The model under review builds one solid part; all positions refer to its coordinate system, in mm. Face numbers are marked on the shaded views. A direction names the side the tool comes from. Coordinates: 2 decimals unless noted, no trailing zeros. Order: outer loops, then holes, each group sorted by start corner. A loop starts at its lowest first (then second) coordinate and runs counter-clockwise, first axis right, second up. Notation, with made-up numbers: (-10.5, 3.5) -> (43.5, 3.5) arc R9 ccw to (43.5, 16.5) -> close; hole circle Ø4 at (6, -8.5). An arc over 180 degrees is marked (long way). Answer as CSV lines item,"result". Start each with the question number.
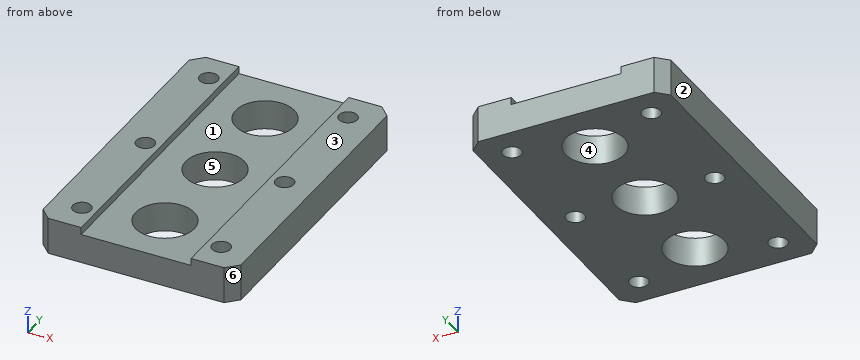
from build123d import *

# Parameters (mm, degrees)
F0_W     = 54
F0_H     = 82
F0_R     = 2.5
F0_R_2   = 8
F1_DEPTH = 10
F2_SIZE  = 3
F3_W     = 30
F3_H     = 82
F4_DEPTH = 2
F5_R     = 8
F6_DEPTH = 25


with BuildPart() as f1:
    # F0 (on Top) → F1 (new body)
    with BuildSketch(Plane.XY):
        Rectangle(F0_W, F0_H)
        with Locations((-19, -33)):
            Circle(F0_R, mode=Mode.SUBTRACT)
        with Locations((0, -26)):
            Circle(F0_R_2, mode=Mode.SUBTRACT)
        with Locations((19, -33)):
            Circle(F0_R, mode=Mode.SUBTRACT)
        with Locations((-19, 0)):
            Circle(F0_R, mode=Mode.SUBTRACT)
        with Locations((-19, 33)):
            Circle(F0_R, mode=Mode.SUBTRACT)
        with Locations((19, 0)):
            Circle(F0_R, mode=Mode.SUBTRACT)
        with Locations((0, 26)):
            Circle(F0_R_2, mode=Mode.SUBTRACT)
        with Locations((19, 33)):
            Circle(F0_R, mode=Mode.SUBTRACT)
    extrude(amount=F1_DEPTH)

    # F2
    f2_edges = [f1.edges().sort_by_distance(p)[0] for p in [
        (27, -41, 5),
        (-27, -41, 5),
        (27, 41, 5),
        (-27, 41, 5),
    ]]
    chamfer(f2_edges, length=F2_SIZE)

    # F3 (on face) → F4 (cut)
    with BuildSketch(Plane.XY.offset(10)):
        Rectangle(F3_W, F3_H)
    extrude(amount=-F4_DEPTH, mode=Mode.SUBTRACT)

    # F5 (on face) → F6 (cut)
    with BuildSketch(Plane.XY.offset(8)):
        Circle(F5_R)
    extrude(amount=-F6_DEPTH, mode=Mode.SUBTRACT)


solid = f1.part
1) Insertion check: pin 1 Ø9.5 at (x, y) = (0, 0) entering from -Z; pin 2 Ø1 at (x, y) = (10.5, 28) entering from +Z. Each pin has a flat end and moves straight along its axis. Give the tip position at first contact, or say it passes through.
2) Consider section B-B (x = -19). Give the boundary of the cut face in (y, z), plus the area to 3 significant figures.
3) Tool access review of the marked faces 1 and 2: name each direction out of +Z, -Z, +X, -X, +Y, -Y from which nothing blocks a thin tool from reaching the whole face with its end or side.
4) Consider section D-D (z = 1). Count the separate pieces of the cut face and the enclosed holes in it, plus the area to 3 significant figures.
5) Consider section C-C (y = -26). Give the boundary of the cut face in (x, z).
6) Mouldability with a two-part tool opening along Y and no side actions: class the marked faces 3, 4, 5 and 6 as released by +Y, released by -Y, zero draft, split by the parting line, or undercut.
7) Consider section A-A (z = 9). Give the boundary of the cut face in (x, y).
8) Wall thickness on L1, parallel to Y at x = -19, z = 2.5; L2, parallel to Y at x = 0, z = 6; L3, parallel to X at y = 26, z = 3.75: over which ranges is each line inside the solid? List them lowest first. Write a range as [from, to].
Result:
1,pin 1,"through"
1,pin 2,"z = 8"
2,outline,"(-41, 0) -> (-35.5, 0) -> (-35.5, 10) -> (-41, 10) -> close; (-30.5, 0) -> (-2.5, 0) -> (-2.5, 10) -> (-30.5, 10) -> close; (2.5, 0) -> (30.5, 0) -> (30.5, 10) -> (2.5, 10) -> close; (35.5, 0) -> (41, 0) -> (41, 10) -> (35.5, 10) -> close"
2,area,"670 mm2"
3,face 1,"+Z, +Y, -Y"
3,face 2,"+Z, -Z, -X, +Y, -Y"
4,separate pieces,"1"
4,enclosed holes,"9"
4,area,"3,690 mm2"
5,outline,"(-27, 0) -> (-8, 0) -> (-8, 8) -> (-15, 8) -> (-15, 10) -> (-27, 10) -> close; (8, 0) -> (27, 0) -> (27, 10) -> (15, 10) -> (15, 8) -> (8, 8) -> close"
6,face 3,"zero draft"
6,face 4,"undercut"
6,face 5,"undercut"
6,face 6,"released by -Y"
7,outline,"(-27, -38) -> (-24, -41) -> (-15, -41) -> (-15, 41) -> (-24, 41) -> (-27, 38) -> close; (15, -41) -> (24, -41) -> (27, -38) -> (27, 38) -> (24, 41) -> (15, 41) -> close; hole circle Ø5 at (-19, -33); hole circle Ø5 at (-19, 0); hole circle Ø5 at (-19, 33); hole circle Ø5 at (19, -33); hole circle Ø5 at (19, 0); hole circle Ø5 at (19, 33)"
8,L1,"[-41, -35.5], [-30.5, -2.5], [2.5, 30.5], [35.5, 41]"
8,L2,"[-41, -34], [-18, -8], [8, 18], [34, 41]"
8,L3,"[-27, -8], [8, 27]"
